Work out the finished part from the listing and answer in its coordinate system (mm). Face numbers are marked on the shaded views. A direction names the side the tool comes from. Coordinates: 2 decimals unless noted, no trailing zeros. Loops run counter-clockwise (first coordinate to the right, second up) from the corner with the lowest first, then second, coordinate; pieces in that order, holes last. Notation, with made-up numbers: (15.25, 21.25) -> (51.25, 21.25) arc R35 cw to (51.25, 56.25) -> close; hole circle Ø3 at (53.5, 79.25). An arc over 180 degrees is marked (long way). Use a Markdown table: item, result.
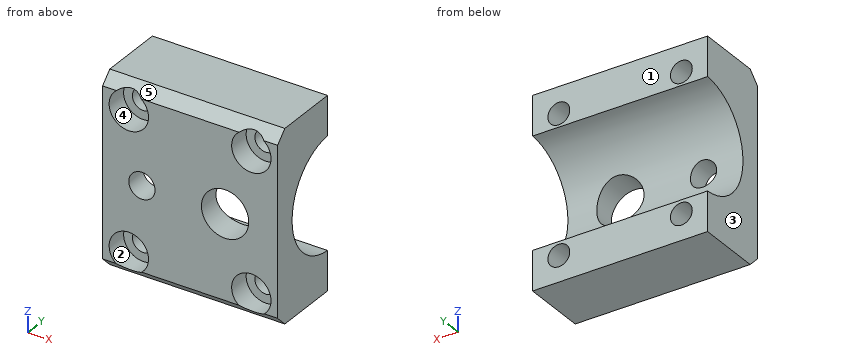
from build123d import *

# Parameters (mm, degrees)
F1_DEPTH       = 40
F3_D           = 5
F3_CBORE_D     = 9
F3_CBORE_DEPTH = 5
F4_T1_DEPTH    = 52.8584149398
F5_R           = 3
F6_DEPTH       = 17.201
F8_D           = 10.8
F8_DEPTH       = 11.35
F8_TIP         = 3.2446473427


# Not quite as in the source:
# - a fillet or chamfer that OpenCascade refuses, or shapes differently, is made with other operations: its cross-section is extruded or revolved along the edge and cut away or added


with BuildPart() as f1:
    # F0 (on Right) → F1 (new body)
    with BuildSketch(Plane.YZ):
        with BuildLine():
            ThreePointArc((-0.5, -12.6901536634), (-12.7, 0), (-0.5, 12.6901536634))
            Line((-0.5, 12.6901536634), (-0.5, 21.7))
            Line((-0.5, 21.7), (-17.7, 21.7))
            Line((-17.7, 21.7), (-17.7, -21.7))
            Line((-17.7, -21.7), (-0.5, -21.7))
            Line((-0.5, -21.7), (-0.5, -12.6901536634))
        make_face()
    extrude(amount=F1_DEPTH)

    # F3 (through all)
    with Locations(Plane.XZ.offset(17.7)):
        with Locations((6, 15.7), (34, 15.7), (34, -15.8), (6, -15.8)):
            CounterBoreHole(F3_D / 2, F3_CBORE_D / 2, F3_CBORE_DEPTH)

    # F4: chamfer of 2.5 on 2 edges, made by hand

    # F4_s2 → F4_t1 (cut)
    with BuildSketch(Plane.YZ.offset(-6.4292074699)):
        Polygon((-15.2, 21.7), (-17.7, 19.2), (-17.7, 21.7), align=None)
        Polygon((-15.2, -21.7), (-17.7, -19.2), (-17.7, -21.7), align=None)
    extrude(amount=F4_T1_DEPTH, mode=Mode.SUBTRACT)

    # F5 (on face) → F6 (cut, through all)
    with BuildSketch(Plane.XZ.offset(17.7)):
        with Locations((9, 0)):
            Circle(F5_R)
    extrude(amount=-F6_DEPTH, mode=Mode.SUBTRACT)

    # F8
    with Locations(Plane.XZ.offset(17.7)):
        with Locations((28, 0)):
            Hole(F8_D / 2, depth=F8_DEPTH)
            with Locations((0, 0, -(F8_DEPTH + F8_TIP / 2))):  # 118° drill point
                Cone(0, F8_D / 2, F8_TIP, mode=Mode.SUBTRACT)


solid = f1.part
Q1. Section C-C on x = 28 is taken. Determine the outline of the cut face in (y, z), and give its area (3 significant figures).
Solved:
| item | result |
|---|---|
| outline | (-17.7, -19.2) -> (-15.2, -21.7) -> (-0.5, -21.7) -> (-0.5, -12.69) arc R12.7 cw to (-11.49, -5.4) -> (-17.7, -5.4) -> close; (-17.7, 5.4) -> (-11.49, 5.4) arc R12.7 cw to (-0.5, 12.69) -> (-0.5, 21.7) -> (-15.2, 21.7) -> (-17.7, 19.2) -> close |
| area | 441 mm² |
Q2. Section D-D on x = 17 is taken. Determine the outline of the cut face in (y, z), and give its area (3 significant figures).
Solved:
| item | result |
|---|---|
| outline | (-17.7, -19.2) -> (-15.2, -21.7) -> (-0.5, -21.7) -> (-0.5, -12.69) arc R12.7 cw to (-0.5, 12.69) -> (-0.5, 21.7) -> (-15.2, 21.7) -> (-17.7, 19.2) -> close |
| area | 500 mm² |
Q3. Consider line 1 (X direction, y = -13.5, z = 15); line 2 (Z direction, x = 28, y = -13); line 3 (X direction, y = -12.5, z = 18). Determine where each line is inside the solid, lowest interval first. Write a range as [from, to].
Solved:
| item | result |
|---|---|
| line 1 | [0, 1.55], [10.45, 29.55], [38.45, 40] |
| line 2 | [-21.7, -5.4], [5.4, 21.7] |
| line 3 | [0, 5.02], [6.98, 33.02], [34.98, 40] |
Q4. Determine the mould class of the marked faces 3, 4 and 5 for opening direction X: pulls with the +X half, pulls with the -X half, needs draft (parallel to the pull), parting line crosses it, or undercut.
Solved:
| item | result |
|---|---|
| face 3 | pulls with the -X half |
| face 4 | undercut |
| face 5 | needs draft |
Q5. Given pin 1 Ø4 at (x, z) = (6, -15.8) entering from +Y; pin 2 Ø7 at (x, z) = (6, 15.7) entering from -Y; pin 3 Ø1.5 at (x, z) = (13, -11) entering from +Y; pin 4 Ø14 at (x, z) = (28, 0) entering from +Y, each flat-ended and moving along its own axis, determine where each tip first touches the part or whether it passes through.
Solved:
| item | result |
|---|---|
| pin 1 | through |
| pin 2 | y = -12.7 |
| pin 3 | y = -4.82 |
| pin 4 | y = -10.6 |
Q6. Section B-B on y = -7.75 is taken. Determine the outline of the cut face in (x, z), and give its area (3 significant figures).
Solved:
| item | result |
|---|---|
| outline | (0, -21.7) -> (40, -21.7) -> (40, -10.06) -> (0, -10.06) -> close; (0, 10.06) -> (40, 10.06) -> (40, 21.7) -> (0, 21.7) -> close; hole circle Ø5 at (6, -15.8); hole circle Ø5 at (6, 15.7); hole circle Ø5 at (34, -15.8); hole circle Ø5 at (34, 15.7) |
| area | 853 mm² |
Q7. Section A-A on z = 0 is taken. Determine the outline of the cut face in (x, y), and give its area (3 significant figures).
Solved:
| item | result |
|---|---|
| outline | (0, -17.7) -> (6, -17.7) -> (6, -12.7) -> (0, -12.7) -> close; (12, -17.7) -> (22.6, -17.7) -> (22.6, -12.7) -> (12, -12.7) -> close; (33.4, -17.7) -> (40, -17.7) -> (40, -12.7) -> (33.4, -12.7) -> close |
| area | 116 mm² |
Q8. For the marked faces 1 and 2, determine the directions among +Z, -Z, +X, -X, +Y, -Y from which every point of the face is accessible in a straight line to the end or side of a thin tool.
Solved:
| item | result |
|---|---|
| face 1 | +Z, -Z, +X, -X, +Y |
| face 2 | -Y |
